Verification items for the finished model (mm, model axes). A direction names the side the tool comes from. Round coordinates to 2 decimals unless told otherwise and drop trailing zeros. Write each loop counter-clockwise with the first axis right and the second up, starting at its lowest first coordinate (ties: lowest second). Pieces come first, ordered by that corner, then holes. Notation, with made-up numbers: M 80,61 L 102,61 A21 cw 102,69 Z; hole C 87.25,-4.5 d2. An arc over 180 degrees is marked long. Use a Markdown table: item, result. Add a question column.
from build123d import *

# Parameters (mm, degrees)
F0_R     = 44.45
F1_DEPTH = 12.7
F2_R     = 28.575
F2_R_2   = 19.05
F3_DEPTH = 38.1
F5_DEPTH = 12.701
F6_R     = 2.5
F7_DEPTH = 44.451
F8_DEPTH = 44.451


with BuildPart() as f1:
    # F0 (on Top) → F1 (new body)
    with BuildSketch(Plane.XY):
        Circle(F0_R)
    extrude(amount=F1_DEPTH)

    # F2 (on face) → F3 (join)
    with BuildSketch(Plane.XY.offset(12.7)):
        Circle(F2_R)
        Circle(F2_R_2, mode=Mode.SUBTRACT)
    extrude(amount=F3_DEPTH)

    # F4 (on face) → F5 (cut, through all)
    with BuildSketch(Plane.XY.offset(12.7)):
        with BuildLine():
            Line((0, -36.5125), (0, -34.0125))
            ThreePointArc((0, -34.0125), (-2.5, -36.5125), (0, -39.0125))
            Line((0, -39.0125), (0, -36.5125))
        make_face()
        with BuildLine():
            ThreePointArc((2.5, -36.5125), (1.767767, -34.744733), (0, -34.0125))
            Line((0, -34.0125), (0, -36.5125))
            Line((0, -36.5125), (0, -39.0125))
            ThreePointArc((0, -39.0125), (1.767767, -38.280267), (2.5, -36.5125))
        make_face()
        with BuildLine():
            ThreePointArc((-39.0125, 0), (-36.5125, -2.5), (-34.0125, 0))
            Line((-34.0125, 0), (-36.5125, 0))
            Line((-36.5125, 0), (-39.0125, 0))
        make_face()
        with BuildLine():
            Line((-36.5125, 0), (-34.0125, 0))
            ThreePointArc((-34.0125, 0), (-36.5125, 2.5), (-39.0125, 0))
            Line((-39.0125, 0), (-36.5125, 0))
        make_face()
        with BuildLine():
            ThreePointArc((0, 39.0125), (-2.5, 36.5125), (0, 34.0125))
            Line((0, 34.0125), (0, 36.5125))
            Line((0, 36.5125), (0, 39.0125))
        make_face()
        with BuildLine():
            Line((34.0125, 0), (36.5125, 0))
            Line((36.5125, 0), (39.0125, 0))
            ThreePointArc((39.0125, 0), (36.5125, 2.5), (34.0125, 0))
        make_face()
        with BuildLine():
            Line((39.0125, 0), (36.5125, 0))
            Line((36.5125, 0), (34.0125, 0))
            ThreePointArc((34.0125, 0), (36.5125, -2.5), (39.0125, 0))
        make_face()
        with BuildLine():
            Line((0, 36.5125), (0, 34.0125))
            ThreePointArc((0, 34.0125), (1.767767, 34.744733), (2.5, 36.5125))
            ThreePointArc((2.5, 36.5125), (1.767767, 38.280267), (0, 39.0125))
            Line((0, 39.0125), (0, 36.5125))
        make_face()
    extrude(amount=-F5_DEPTH, mode=Mode.SUBTRACT)

    # F6 (on Front) → F7 (cut, through all)
    with BuildSketch(Plane.XZ):
        with Locations((0, 25.549719)):
            Circle(F6_R)
    extrude(amount=-F7_DEPTH, mode=Mode.SUBTRACT)

    # F6 (on Front) → F8 (cut, through all)
    with BuildSketch(Plane.XZ):
        with Locations((0, 25.549719)):
            Circle(F6_R)
    extrude(amount=F8_DEPTH, mode=Mode.SUBTRACT)


solid = f1.part
1. Depth check by flat-ended pin: pin 1 Ø8 at (x, z) = (-4, 15) entering from -Y; pin 2 Ø12 at (y, z) = (-13.5, 6.5) entering from +X; pin 3 Ø1 at (x, y) = (5.5, -2.5) entering from +Z. Enter the tip coordinate at first touch or a pass-through.
2. Cross-section at B-B on z = 5.5. Enter the section's corners in (x, y), plus the area to 3 significant figures.
3. Scan lines: line 1 along Z through (x, y) = (0, -25.75); line 2 along Y through (x, z) = (0, 29.5) (3 decimals); line 3 along Y through (x, z) = (5, 18). Record each from-to range of solid material in increasing order. Write a range as from..to.
4. Cross-section at A-A on y = 0. Count the separate pieces of the cut face and the enclosed holes in it, plus the area to 3 significant figures.
5. Release check for a two-part mould opening along Y. For faces 1 (the cylindrical face through (42.397, 13.352, 6.261)), 2 (the cylindrical face through (34.203, 0.958, 6.439)), 3 (the flat face through (6, -19, 50.8)) record: +Y half, -Y half, draft (parallel to the pull), parting line (faces both ways), or undercut.
6. Access from +Z, -Z, +X, -X, +Y, -Y to the whole of each face (thin tool, end or side, straight path). Record for faces 4 (the flat face through (-1, 1, 0)), 5 (the cylindrical face through (-28.547, 1.256, 31.483)).
7. Cross-section at C-C on z = 42. Enter the section's corners in (x, y) (3 decimals).
8. Cross-section at D-D on x = 8. Enter the section's corners in (y, z), plus the area to 3 significant figures.
Answer:
| question | item | result |
|---|---|---|
| 1 | pin 1 | stops at y = -44.44 |
| 1 | pin 2 | stops at x = 43.81 |
| 1 | pin 3 | stops at z = 12.7 |
| 2 | outline | C 0,0 d88.9; hole C -36.51,0 d5; hole C 0,-36.51 d5; hole C 0,36.51 d5; hole C 36.51,0 d5 |
| 2 | area | 6,130 mm^2 |
| 3 | line 1 | z = 0..23.05, 28.05..50.8 |
| 3 | line 2 | y = -28.575..-19.05, 19.05..28.575 |
| 3 | line 3 | y = -28.13..-18.38, 18.38..28.13 |
| 4 | separate pieces | 3 |
| 4 | enclosed holes | 0 |
| 4 | area | 1,730 mm^2 |
| 5 | face 1 | parting line |
| 5 | face 2 | undercut |
| 5 | face 3 | draft |
| 6 | face 4 | -Z, +X, -X, +Y, -Y |
| 6 | face 5 | +Z |
| 7 | outline | C 0,0 d57.15; hole C 0,0 d38.1 |
| 8 | outline | M -43.72,0 L 43.72,0 L 43.72,12.7 L 27.43,12.7 L 27.43,50.8 L 17.29,50.8 L 17.29,12.7 L -17.29,12.7 L -17.29,50.8 L -27.43,50.8 L -27.43,12.7 L -43.72,12.7 Z |
| 8 | area | 1,880 mm^2 |
